from build123d import *

# Parameters (mm, degrees)
SKETCH001_R     = 4.5
SKETCH001_R_2   = 3
PAD001_DEPTH    = 3
CHAMFER_SIZE    = 0.5
SKETCH002_R     = 7.4
SKETCH002_R_2   = 4.5
PAD002_DEPTH    = 3
CHAMFER001_SIZE = 0.5
SKETCH_R        = 8.5
SKETCH_R_2      = 7.4
PAD_DEPTH       = 3
CHAMFER002_SIZE = 0.2


with BuildPart() as innerrace:
    # Sketch001 → Pad001 (new body, symmetric)
    with BuildSketch(Plane.XY):
        Circle(SKETCH001_R)
        Circle(SKETCH001_R_2, mode=Mode.SUBTRACT)
    extrude(amount=PAD001_DEPTH, both=True)

    # Chamfer
    chamfer_edges = [innerrace.edges().sort_by_distance(p)[0] for p in [
        (-4.5, 0, 3),
        (-3, 0, 3),
        (-4.5, 0, -3),
        (-3, 0, -3),
    ]]
    chamfer(chamfer_edges, length=CHAMFER_SIZE)


with BuildPart() as seal:
    # Sketch002 → Pad002 (new body, symmetric)
    with BuildSketch(Plane.XY):
        Circle(SKETCH002_R)
        Circle(SKETCH002_R_2, mode=Mode.SUBTRACT)
    extrude(amount=PAD002_DEPTH, both=True)

    # Chamfer001
    chamfer001_edges = [seal.edges().sort_by_distance(p)[0] for p in [
        (-7.4, 0, -3),
        (-4.5, 0, -3),
        (-7.4, 0, 3),
        (-4.5, 0, 3),
    ]]
    chamfer(chamfer001_edges, length=CHAMFER001_SIZE)


with BuildPart() as fusion:
    # Sketch → Pad (new body, symmetric)
    with BuildSketch(Plane.XY):
        Circle(SKETCH_R)
        Circle(SKETCH_R_2, mode=Mode.SUBTRACT)
    extrude(amount=PAD_DEPTH, both=True)

    # Chamfer002
    chamfer002_edges = [fusion.edges().sort_by_distance(p)[0] for p in [
        (8.5, 0, 0),
        (-8.5, 0, -3),
        (-8.5, 0, 3),
    ]]
    chamfer(chamfer002_edges, length=CHAMFER002_SIZE)

    # Fusion: union InnerRace, Seal
    add(innerrace.part)
    add(seal.part)


solid = fusion.part
Model file for the job. Use its own axes, mm. Round coordinates to 2 decimals unless told otherwise and drop trailing zeros. Order: outer loops, then holes, each group sorted by start corner. A loop starts at its lowest first (then second) coordinate and runs counter-clockwise, first axis right, second up.
(1) Drill centre lines: line 1 (Y direction, x = 0, z = -0.6); line 2 (Y direction, x = 5.75, z = 2.65); line 3 (Y direction, x = -0.75, z = 0.6). Where is each one in solid material? Low to high.
(2) Pull direction Y, two halves, no side cores. Call faces 1 (the face through (4.57, 7.167, 0.039)), 2 (the face through (-6, -5, 3)), 3 (the face through (-3, 0, 0)), 4 (the face through (-1.604, -7.224, -2.754)): released by +Y, released by -Y, zero draft, split by the parting line, or undercut.
(3) Pin check, flat tip, straight feed: pin 1 (3 mm diameter, centred on y = -6.5, z = 2, fed in from -X). Stop position of the tip, or through.
(4) Band-saw the part on A-A (z = 0.1). List the corners of the cut face in (x, y).
Verdict:
1. line 1: y = -8.5 to -3, 3 to 8.5
1. line 2: y = -6.26 to -4.66, -4.42 to 4.42, 4.66 to 6.26
1. line 3: y = -8.47 to -2.9, 2.9 to 8.47
2. face 1: split by the parting line
2. face 2: zero draft
2. face 3: undercut
2. face 4: undercut
3. pin 1: stops at x = -6.87
4. outline: circle Ø17 at (0, 0); hole circle Ø6 at (0, 0)
